Source: three-view drawing plus pictorial views. Frame: mm from the lowest corner of the part. Coordinates: 2 decimals unless noted, no trailing zeros. Loops run counter-clockwise (first coordinate to the right, second up) from the corner with the lowest first, then second, coordinate; pieces in that order, holes last. Notation, with made-up numbers: (0.5, -33) -> (33.5, -33) arc R15 ccw to (33.5, -16) -> close; hole circle Ø4 at (24.5, 39). An arc over 180 degrees is marked (long way). Answer as a JSON object with one key per item and string values. Group by question number.
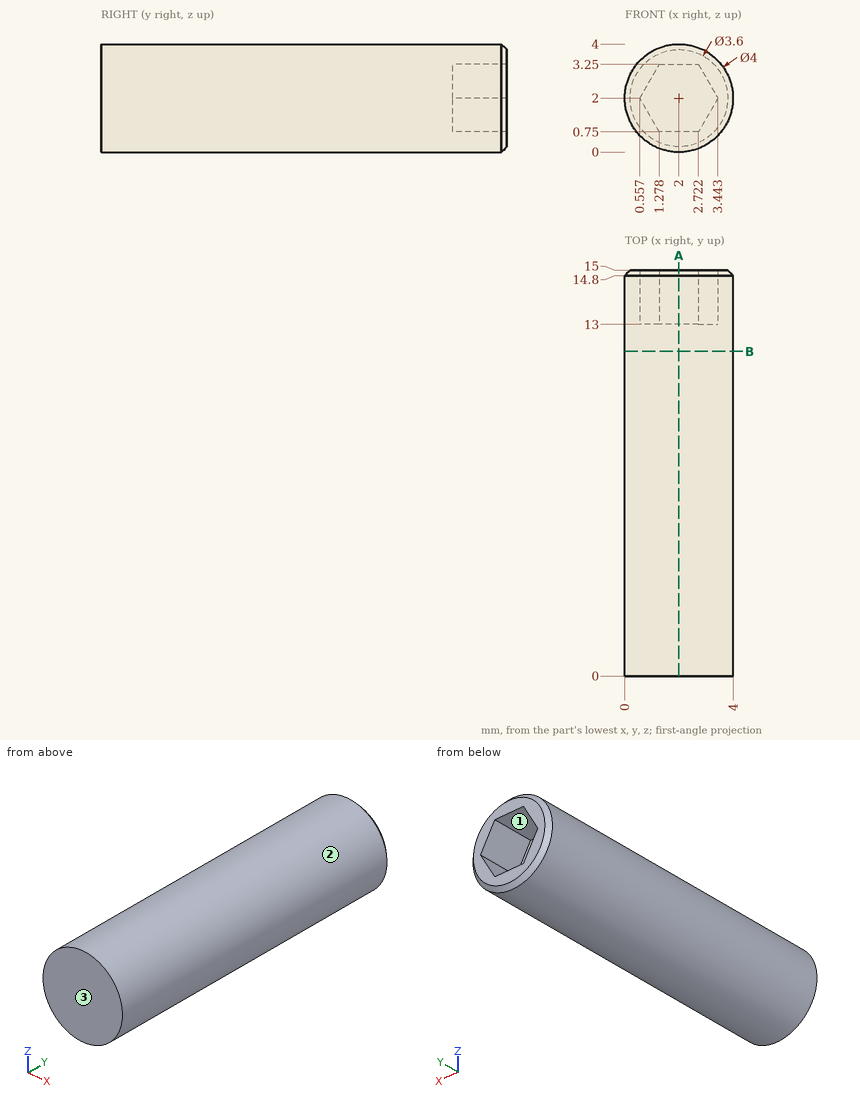
1. Mould query, pull axis X, two halves, no side actions, for the marked faces 1, 2 and 3. Classes: pulls with the +X half, pulls with the -X half, needs draft (parallel to the pull), parting line crosses it, or undercut.
2. Section query A-A on x = 2. Return loops of the section in (y, z).
3. Section query B-B on y = 12. Return loops of the section in (x, z).
4. Ray query, L1, parallel to Y at x = 2.2, z = 1.35; L2, parallel to X at y = 14.75, z = 1.2; L3, parallel to Z at x = 1.05, y = 10. Return the intervals inside material, ascending.
Solved:
{
 "1": {"face 1": "undercut", "face 2": "parting line crosses it", "face 3": "needs draft"},
 "2": {"outline": "(0, 0) -> (14.8, 0) -> (15, 0.2) -> (15, 0.75) -> (13, 0.75) -> (13, 3.25) -> (15, 3.25) -> (15, 3.8) -> (14.8, 4) -> (0, 4) -> close"},
 "3": {"outline": "circle Ø4 at (2, 2)"},
 "4": {"L1": "0 to 13", "L2": "0.17 to 1.02, 2.98 to 3.83", "L3": "0.24 to 3.76"}
}
